Build history of the part. All positions in model axes, mm. Round coordinates to 2 decimals unless told otherwise and drop trailing zeros. Write each loop counter-clockwise with the first axis right and the second up, starting at its lowest first coordinate (ties: lowest second). Pieces come first, ordered by that corner, then holes. Notation, with made-up numbers: (-14, 29) -> (14, 29) arc R10 ccw to (14, 33) -> close; hole circle Ø10 at (51, 81). An arc over 180 degrees is marked (long way). Answer in a Markdown table with one row per item.
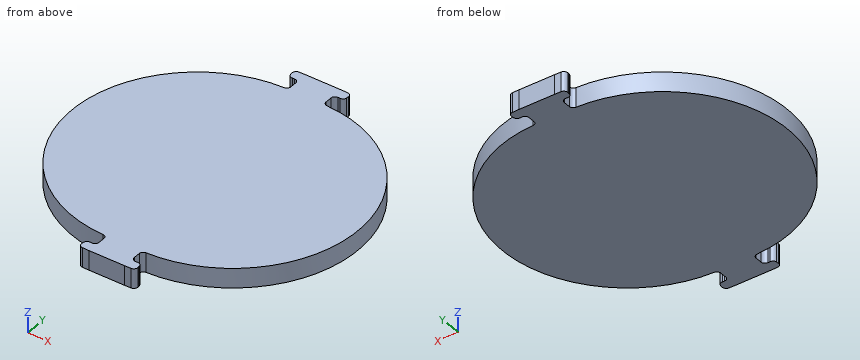
```python
from build123d import *

# Parameters (mm, degrees)
F1_DEPTH = 6.35
F2_R     = 1.27


with BuildPart() as f1:
    # F0 (on Top) → F1 (new body)
    with BuildSketch(Plane.XY):
        with BuildLine():
            Line((0, -40.48125), (0, -41.275))
            Line((0, -41.275), (0, -41.28198))
            Line((0, -41.28198), (0, -45.24375))
            ThreePointArc((0, -45.24375), (-1.616893, -45.209426), (-3.230874, -45.106514))
            Line((-3.230874, -45.106514), (-3.500113, -48.270078))
            ThreePointArc((-3.500113, -48.270078), (-1.751635, -48.381565), (0, -48.41875))
            Line((0, -48.41875), (11.43, -48.41875))
            ThreePointArc((11.43, -48.41875), (13.181635, -48.381565), (14.930113, -48.270078))
            Line((14.930113, -48.270078), (14.660874, -45.106514))
            ThreePointArc((14.660874, -45.106514), (13.046893, -45.209426), (11.43, -45.24375))
            Line((11.43, -45.24375), (11.43, -40.48125))
            ThreePointArc((11.43, -40.48125), (51.91125, 0), (11.43, 40.48125))
            Line((11.43, 40.48125), (11.43, 45.24375))
            ThreePointArc((11.43, 45.24375), (13.046893, 45.209426), (14.660874, 45.106514))
            Line((14.660874, 45.106514), (14.930113, 48.270078))
            ThreePointArc((14.930113, 48.270078), (13.181635, 48.381565), (11.43, 48.41875))
            Line((11.43, 48.41875), (0, 48.41875))
            ThreePointArc((0, 48.41875), (-1.751635, 48.381565), (-3.500113, 48.270078))
            Line((-3.500113, 48.270078), (-3.230874, 45.106514))
            ThreePointArc((-3.230874, 45.106514), (-1.616893, 45.209426), (0, 45.24375))
            Line((0, 45.24375), (0, 41.275))
            Line((0, 41.275), (0, 41.207306))
            Line((0, 41.207306), (0, 40.48125))
            ThreePointArc((0, 40.48125), (-40.48125, 0), (0, -40.48125))
        make_face()
    extrude(amount=F1_DEPTH)

    # F2
    f2_edges = [f1.edges().sort_by_distance(p)[0] for p in [
        (0, -40.48125, 3.175),
        (11.43, -40.48125, 3.175),
        (14.930113, -48.270078, 3.175),
        (14.660874, -45.106514, 3.175),
        (-3.500113, -48.270078, 3.175),
        (-3.230874, -45.106514, 3.175),
        (14.660874, 45.106514, 3.175),
        (14.930113, 48.270078, 3.175),
        (-3.500113, 48.270078, 3.175),
        (-3.230874, 45.106514, 3.175),
        (0, 45.24375, 3.175),
        (0, 40.48125, 3.175),
        (11.43, -45.24375, 3.175),
        (0, -45.24375, 3.175),
        (11.43, 40.48125, 3.175),
        (11.43, 45.24375, 3.175),
    ]]
    fillet(f2_edges, radius=F2_R)


solid = f1.part
```
Q1. Saw through at A-A on x = 38. Write the cut outline in (y, z), plus the area to 3 significant figures.
A:
| item | result |
|---|---|
| outline | (-30.54, 0) -> (30.54, 0) -> (30.54, 6.35) -> (-30.54, 6.35) -> close |
| area | 388 mm² |
Q2. Drop flat-ended pins along their axis: P1, Ø2.5, axis at y = 42.5, z = 4.5, coming from the +X side (3 decimals); P2, Ø2.5, axis at y = 43, z = 3.5, coming from the -X side; P3, Ø2.5, axis at y = -42.5, z = 2, coming from the -X side (3 decimals). Give the stop position or say it passes through.
A:
| item | result |
|---|---|
| P1 | x = 11.525 |
| P2 | x = -0.04 |
| P3 | x = -0.095 |
Q3. Saw through at B-B on y = -17.5. Write the cut outline in (x, z).
A:
| item | result |
|---|---|
| outline | (-36.5, 0) -> (47.93, 0) -> (47.93, 6.35) -> (-36.5, 6.35) -> close |
Q4. Wall check: line 1 (X direction, y = 29, z = 2.5); line 2 (X direction, y = -24, z = 2.25); line 3 (Y direction, x = 42, z = 2.25). Give the ranges that are in metal, low to high. Write a range as [from, to].
A:
| item | result |
|---|---|
| line 1 | [-28.24, 39.67] |
| line 2 | [-32.6, 44.03] |
| line 3 | [-26.54, 26.54] |
